Autodesk Inventor part; units mm, degrees
ref_plane "YZ Plane" through (0, 0, 0) normal (1, 0, 0) x (0, 1, 0)
ref_plane "XZ Plane" through (0, 0, 0) normal (0, 1, 0) x (-1, 0, 0)
ref_plane "XY Plane" through (0, 0, 0) normal (0, 0, 1) x (1, 0, 0)
sketch "Sketch1" plane through (0, 0, 0) normal (0, 0, 1) x (1, 0, 0)
  line L0 (0, 3.5) -> (0, -3.5)
  line L1 (0, -3.5) -> (0.75, -3.5)
  line L2 (0.75, -3.5) -> (1, -3.25)
  line L3 (1, -3.25) -> (1, 1.4)
  line L4 (1.1, 1.5) -> (1.65, 1.5)
  line L5 (1.9, 1.75) -> (1.9, 3.25)
  line L6 (1.65, 3.5) -> (0, 3.5)
  arc A0 (1.1, 1.5) -> (1, 1.4) centre (1.1, 1.4) ccw
  line L7 (1.65, 3.5) -> (1.9, 3.25)
  line L8 (1.65, 1.5) -> (1.9, 1.75)
  point P0 (0, 0)
  point P1 (1.9, 1.5)
  point P2 (1.9, 3.5)
  point P3 (0, 0)
  dimension "d0" = 3.8
  dimension "d1" = 2
  dimension "d3" = 2
  dimension "d4" = 2.2
  dimension "d5" = 135
  dimension "d6" = 0.25
  dimension "d7" = 5
  dimension "d18" = 0.25
revolve "Revolution1" add sketch "Sketch1" angle 360 about axis through (0, 3.5, 0) along (0, -1, 0)
sketch "Sketch2" plane through (0, 3.5, 0) normal (0, 1, 0) x (1, 0, 0)
  line L0 (0, -0.866) -> (-0.75, -0.433)
  line L1 (-0.75, -0.433) -> (-0.75, 0.433)
  line L2 (-0.75, 0.433) -> (0, 0.866)
  line L3 (0, 0.866) -> (0.75, 0.433)
  line L4 (0.75, 0.433) -> (0.75, -0.433)
  line L5 (0.75, -0.433) -> (0, -0.866)
  point P0 (0, 0)
  point P1 (0, 0)
  dimension "d11" = 1.5
extrude "Extrusion1" cut sketch "Sketch2" against normal blind 1.5
thread "Thread1"
sketch "Sketch3" plane through (0, 0, 0) normal (1, 0, 0) x (0, 1, 0)
  line L0 (3.5, 0.866) -> (3.5, 0.433)
  line L1 (3.5, 0.866) -> (3, 0.366)
  line L2 (3, 0.366) -> (3.5, 0.366)
  line L3 (3.5, 0.366) -> (3.5, 0.866)
  line L4 (-0.6, 0) -> (3.6, 0)
  point P0 (0, 0)
  dimension "d16" = 0.5
revolve "Revolution2" cut sketch "Sketch3" angle 360 about axis through (0, -10, 0) along (0, 1, 0)
properties part number "Bolt_M2x0.4_5mm_SH" material "Stainless Steel"
Can you work these out from the model? Positions are in its coordinate system, mm. A direction names the side the tool comes from. Coordinates: 2 decimals unless noted, no trailing zeros. Loops run counter-clockwise (first coordinate to the right, second up) from the corner with the lowest first, then second, coordinate; pieces in that order, holes last. Notation, with made-up numbers: (81.5, 82) - (85.5, 82) arc R27 ccw to (85.5, 115) - close; hole circle Ø11 at (-32.5, 36.25). An arc over 180 degrees is marked (long way). Answer as a JSON object with one key per item and string values. Group by question number.
Item 1: For pin 1 (1.5 mm diameter, centred on y = -1.5, z = 0, fed in from -X); pin 2 (1.5 mm diameter, centred on y = 2, z = 1, fed in from +X), each with a flat end and sliding along its axis, tell me the tip position at first contact or that it passes through.
Item 2: If we mould it in two halves opening along X, with no side actions, what happens to faces 3 (the face through (0, -3.5, 0)), 4 (the face through (-0.75, 3, 0)), 5 (the face through (0, -1, 1))? For each: released by +X, released by -X, zero draft, split by the parting line, or undercut.
Item 3: On a 3-axis mill with a long thin cutter (end or side, diameter ignored), from which of +Z, -Z, +X, -X, +Y, -Y can I reach the whole of each face in a straight line? I mean faces 1 (the face through (0, 2, 0)), 2 (the face through (1, 3.5, -1)). Say none if no direction works.
Item 4: If we section it at A-A (y = 2.25): List the corners of the cut face in (x, z) for me.
Item 5: If we section it at B-B (z = 0): List the corners of the cut face in (x, y) for me, plus the area to 3 significant figures.
Item 6: If I drill on L1, parallel to X at y = 2.5, z = -0.05; L2, parallel to Y at x = -0.4, z = 1.25; L3, parallel to X at y = -0.25, z = -0.9, over which ranges is the centre line in solid material (lowest first)? Write a range as from..to.
Item 7: If we section it at C-C (y = -1.5): List the corners of the cut face in (x, z) for me, plus the area to 3 significant figures.
Returned:
{
 "1": {"pin 1": "stops at x = -1", "pin 2": "stops at x = 1.88"},
 "2": {"face 3": "zero draft", "face 4": "undercut", "face 5": "split by the parting line"},
 "3": {"face 1": "+Y", "face 2": "+Z, -Z, +X, -X, +Y"},
 "4": {"outline": "circle Ø3.8 at (0, 0); hole (-0.75, -0.43) - (0, -0.87) - (0.75, -0.43) - (0.75, 0.43) - (0, 0.87) - (-0.75, 0.43) - close"},
 "5": {"outline": "(-1.9, 1.75) - (-1.65, 1.5) - (-1.1, 1.5) arc R0.1 cw to (-1, 1.4) - (-1, -3.25) - (-0.75, -3.5) - (0.75, -3.5) - (1, -3.25) - (1, 1.4) arc R0.1 cw to (1.1, 1.5) - (1.65, 1.5) - (1.9, 1.75) - (1.9, 3.25) - (1.65, 3.5) - (0.87, 3.5) - (0.75, 3.38) - (0.75, 2) - (-0.75, 2) - (-0.75, 3.38) - (-0.87, 3.5) - (-1.65, 3.5) - (-1.9, 3.25) - close", "area": "15.2 mm²"},
 "6": {"L1": "x = -1.9..-0.75, 0.75..1.9", "L2": "y = 1.5..3.5", "L3": "x = -0.44..0.44"},
 "7": {"outline": "circle Ø2 at (0, 0)", "area": "3.14 mm²"}
}
